Source: CAD feature listing. Evaluate the final solid. Frame: model axes, mm. Face numbers are marked on the shaded views. A direction names the side the tool comes from. Round coordinates to 2 decimals unless told otherwise and drop trailing zeros. Loops run counter-clockwise (first coordinate to the right, second up) from the corner with the lowest first, then second, coordinate; pieces in that order, holes last. Notation, with made-up numbers: (83, -5.75) - (98, -5.75) arc R16 ccw to (98, 17.25) - close; hole circle Ø9 at (-22, -10.75). An arc over 180 degrees is marked (long way). Write item = value, one per line. Start each with the question number.
Autodesk Inventor part; units mm, degrees
ref_plane "YZ Plane" through (0, 0, 0) normal (1, 0, 0) x (0, 1, 0)
ref_plane "XZ Plane" through (0, 0, 0) normal (0, 1, 0) x (-1, 0, 0)
ref_plane "XY Plane" through (0, 0, 0) normal (0, 0, 1) x (1, 0, 0)
sketch "Sketch1" plane through (0, 0, 0) normal (0, 1, 0) x (-1, 0, 0)
  circle A0 centre (0, 0) radius 26.725
  dimension "d0" = 53.45
extrude "Extrusion1" add sketch "Sketch1" along normal blind 3
sketch "Sketch2" plane through (0, 3, 0) normal (0, 1, 0) x (1, 0, 0)
  circle A0 centre (0, 0) radius 28.8
  dimension "d3" = 57.6
extrude "Extrusion2" add sketch "Sketch2" along normal blind 5.8
sketch "Sketch4" plane through (0, 8.8, 0) normal (0, 1, 0) x (1, 0, 0)
  circle A0 centre (0, 0) radius 31.65
  circle A1 centre (0, 0) radius 28.8
  circle A2 centre (0, 0) radius 28.8
  line L0 (6.3178, -28.0985) -> (-6.3178, -28.0985)
  line L1 (-6.3178, -28.0985) -> (-6.3178, -31.013)
  line L2 (6.3178, -28.0985) -> (6.3178, -31.013)
  line L3 (-6.3178, 28.0985) -> (6.3178, 28.0985)
  line L4 (6.3178, 28.0985) -> (6.3178, 31.013)
  line L5 (-6.3178, 28.0985) -> (-6.3178, 31.013)
  dimension "d13" = 63.3
  dimension "d16" = 360
  dimension "d18" = 56.197
extrude "Extrusion3" add sketch "Sketch4" against normal up to surface (5.8 mm away) contours L4 A1 L5 A0 | A0 L1 A1 L2
fillet "Fillet1" radius 1.4575 8 edges at (-6.3178, 5.9, 28.0985) (-6.3178, 5.9, 31.013) (6.3178, 5.9, 31.013) (6.3178, 5.9, 28.0985) (6.3178, 5.9, -28.0985) (6.3178, 5.9, -31.013) (-6.3178, 5.9, -28.0985) (-6.3178, 5.9, -31.013)
properties part number "HSI cap"
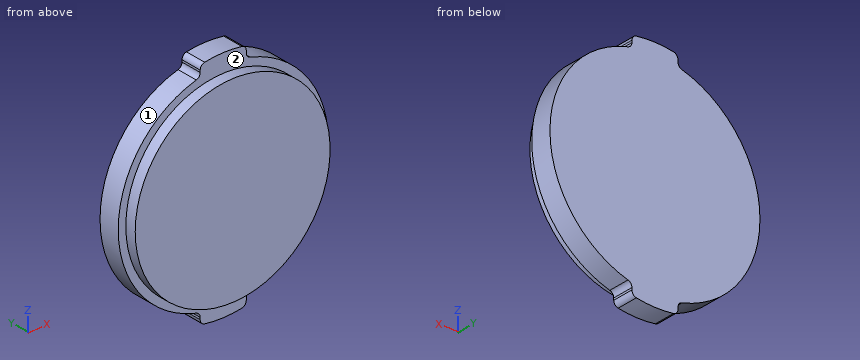
(1) Access query for the marked faces 1 and 2. Directions: +Z, -Z, +X, -X, +Y, -Y. A direction counts if a zero-diameter tool reaches every point of the face in a straight line with its end or side. Return the directions, or none.
(2) Cut plane C-C (y = 1). Output: boundary loops of the cut face in (x, z) (3 decimals), and give its area (3 significant figures).
(3) Material intervals for line 1 along Z through (x, y) = (-5, 5.25); line 2 along X through (y, z) = (4, -9); line 3 along Y through (x, z) = (1, -27.5), sorted ascending. Write a range as from..to.
(4) Cut plane B-B (x = 0). Output: boundary loops of the cut face in (y, z) (3 decimals).
(5) Pin query (flat end, axial travel): P1, Ø5, axis at x = -4.5, y = 3.5, coming from the +Z side; P2, Ø3, axis at y = 4.5, z = 17.5, coming from the -X side; P3, Ø5, axis at x = 12.5, y = 2, coming from the +Z side. Return the tip coordinate at first contact, or that it passes through.
(6) Cut plane A-A (z = 0). Output: boundary loops of the cut face in (x, y) (3 decimals).
Solution:
q1.face_1 = -X, +Y, -Y
q1.face_2 = -Y
q2.outline = circle Ø53.45 at (0, 0)
q2.area = 2,240 mm^2
q3.line_1 = -31.25..31.25
q3.line_2 = -27.36..27.36
q3.line_3 = 3..8.8
q4.outline = (0, -26.725) - (3, -26.725) - (3, -31.65) - (8.8, -31.65) - (8.8, 31.65) - (3, 31.65) - (3, 26.725) - (0, 26.725) - close
q5.P1 = 31.59
q5.P2 = -23.95
q5.P3 = 26.93
q6.outline = (-28.8, 3) - (-26.725, 3) - (-26.725, 0) - (26.725, 0) - (26.725, 3) - (28.8, 3) - (28.8, 8.8) - (-28.8, 8.8) - close
